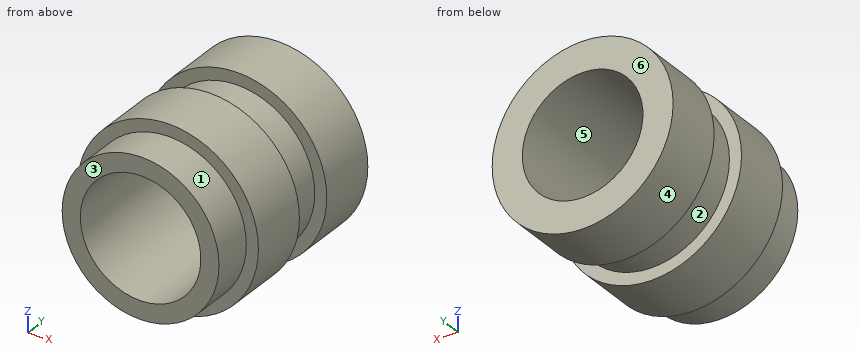
Autodesk Inventor part; units mm, degrees
ref_plane "YZ Plane" through (0, 0, 0) normal (1, 0, 0) x (0, 1, 0)
ref_plane "XZ Plane" through (0, 0, 0) normal (0, 1, 0) x (-1, 0, 0)
ref_plane "XY Plane" through (0, 0, 0) normal (0, 0, 1) x (1, 0, 0)
sketch "Boceto1" plane through (0, 0, 0) normal (0, 1, 0) x (-1, 0, 0)
  circle A0 centre (0, 0) radius 1.95
  dimension "d0" = 3.9
extrude "Extrusión1" add sketch "Boceto1" along normal blind 1
sketch "Boceto2" plane through (0, 1, 0) normal (0, 1, 0) x (1, 0, 0)
  circle A0 centre (0, 0) radius 2.25
  dimension "d3" = 4.5
extrude "Extrusión2" add sketch "Boceto2" along normal blind 1.5
sketch "Boceto3" plane through (0, 2.5, 0) normal (0, 1, 0) x (1, 0, 0)
  circle A0 centre (0, 0) radius 1.95
  dimension "d8" = 3.9
extrude "Extrusión3" add sketch "Boceto3" along normal blind 1
sketch "Boceto4" plane through (0, 3.5, 0) normal (0, 1, 0) x (1, 0, 0)
  circle A0 centre (0, 0) radius 2.25
  circle A1 centre (0, 0) radius 2.25
extrude "Extrusión4" add sketch "Boceto4" along normal blind 1.5
sketch "Boceto5" plane through (0, 5, 0) normal (0, 1, 0) x (1, 0, 0)
  point P0 (0, 0)
  point P1 (0, 0)
hole "Agujero1" at (0, 5, 0) direction (0, -1, 0) diameter 3 depth 6
thread "Rosca1"
properties part number "InsertoM3" material "Latón, amarillo claro"
Verification items for the finished model (mm, model axes). Face numbers are marked on the shaded views. A direction names the side the tool comes from. Give positions to 0.01 mm unless a question says otherwise; leave off trailing zeros. Order: outer loops, then holes, each group sorted by start corner. A loop starts at its lowest first (then second) coordinate and runs counter-clockwise, first axis right, second up. Notation, with made-up numbers: (-18, 11) -> (38, 11) arc R33 cw to (38, 39) -> close; hole circle Ø8 at (83.5, 45.5). An arc over 180 degrees is marked (long way). One line per item, written item: value.
(1) Sectioned sample at C-C on y = 2.4. Record the cut outline in (x, z).
Final values:
outline: circle Ø4.5 at (0, 0); hole circle Ø3 at (0, 0)
(2) Sectioned sample at B-B on x = 0. Record the cut outline in (y, z), then the cut area to 3 significant figures.
Final values:
outline: (0, -1.95) -> (1, -1.95) -> (1, -2.25) -> (2.5, -2.25) -> (2.5, -1.95) -> (3.5, -1.95) -> (3.5, -2.25) -> (5, -2.25) -> (5, -1.5) -> (0, -1.5) -> close; (0, 1.5) -> (5, 1.5) -> (5, 2.25) -> (3.5, 2.25) -> (3.5, 1.95) -> (2.5, 1.95) -> (2.5, 2.25) -> (1, 2.25) -> (1, 1.95) -> (0, 1.95) -> close
area: 6.30 mm^2
(3) Sectioned sample at D-D on x = -1.85. Record the cut outline in (y, z), then the cut area to 3 significant figures.
Final values:
outline: (0, -0.62) -> (1, -0.62) -> (1, -1.28) -> (2.5, -1.28) -> (2.5, -0.62) -> (3.5, -0.62) -> (3.5, -1.28) -> (5, -1.28) -> (5, 1.28) -> (3.5, 1.28) -> (3.5, 0.62) -> (2.5, 0.62) -> (2.5, 1.28) -> (1, 1.28) -> (1, 0.62) -> (0, 0.62) -> close
area: 10.1 mm^2
(4) Sectioned sample at A-A on z = 0. Record the cut outline in (x, y), then the cut area to 3 significant figures.
Final values:
outline: (-2.25, 1) -> (-1.95, 1) -> (-1.95, 0) -> (-1.5, 0) -> (-1.5, 5) -> (-2.25, 5) -> (-2.25, 3.5) -> (-1.95, 3.5) -> (-1.95, 2.5) -> (-2.25, 2.5) -> close; (1.5, 0) -> (1.95, 0) -> (1.95, 1) -> (2.25, 1) -> (2.25, 2.5) -> (1.95, 2.5) -> (1.95, 3.5) -> (2.25, 3.5) -> (2.25, 5) -> (1.5, 5) -> close
area: 6.30 mm^2
(5) Gauge pin test, flat ends, axial feed: pin 1 (2 mm diameter, centred on y = 3, z = -1, fed in from +X); pin 2 (2 mm diameter, centred on x = -1.5, y = 3, fed in from -Z). Record the tip position at first contact, or that the pin passes through.
Final values:
pin 1: x = 2.25
pin 2: z = -2.16
(6) Tool access check on the marked faces 1, 2 and 3. Record the directions out of +Z, -Z, +X, -X, +Y, -Y that give a thin tool (end or side, any length) a straight path to the whole face; none if there is none.
Final values:
face 1: -Y
face 2: none
face 3: +Z, -Z, +X, -X, -Y
(7) Scan lines: line 1 along Z through (x, y) = (0.05, 2.4); line 2 along Y through (x, z) = (1.05, 1.75). Record each from-to range of solid material in increasing order. Write a range as [from, to].
Final values:
line 1: [-2.25, -1.5], [1.5, 2.25]
line 2: [1, 2.5], [3.5, 5]
(8) Draft check along Z on the marked faces 4, 5 and 6. Enter one of: pulls with the +Z half, pulls with the -Z half, needs draft (parallel to the pull), parting line crosses it, or undercut.
Final values:
face 4: parting line crosses it
face 5: undercut
face 6: needs draft
